from build123d import *

# Parameters (mm, degrees)
F0_W            = 304.8
F0_H            = 106.68
F1_DEPTH        = 3.81
F2_W            = 294.132
F2_H            = 96.012
F3_DEPTH        = 2.54
F4_W            = 5.334
F4_H            = 5.334
F4_W_2          = 5.08
F4_H_2          = 5.08
F5_DEPTH        = 25.4
F6_R            = 5.08
F7_DEPTH        = 27.94
F9_DEPTH        = 27.94
F10_D           = 2.032
F10_DEPTH       = 12.7
F10_CSINK_D     = 3.81
F10_CSINK_ANGLE = 90
F10_TIP         = 0.6104743889


with BuildPart() as f1:
    # F0 (on Top) → F1 (new body)
    with BuildSketch(Plane.XY):
        with Locations((152.4, -53.34)):
            Rectangle(F0_W, F0_H)
    extrude(amount=F1_DEPTH)

    # F2 (on face) → F3 (join)
    with BuildSketch(Plane.XY.offset(3.81)):
        with Locations((152.4, -53.34)):
            Rectangle(F2_W, F2_H)
    extrude(amount=F3_DEPTH)

    # F4 (on face) → F5 (join)
    with BuildSketch(Plane.XY.offset(6.35)):
        with Locations((8.001, -8.001)):
            Rectangle(F4_W, F4_H)
        with Locations((8.001, -98.679)):
            Rectangle(F4_W, F4_H)
        with Locations((296.799, -8.001)):
            Rectangle(F4_W, F4_H)
        with Locations((296.799, -98.679)):
            Rectangle(F4_W, F4_H)
        with Locations((152.4, -7.874)):
            Rectangle(F4_W_2, F4_H_2)
        with Locations((152.4, -98.806)):
            Rectangle(F4_W_2, F4_H_2)
    extrude(amount=F5_DEPTH)

    # F6
    f6_edges = [f1.edges().sort_by_distance(p)[0] for p in [
        (294.132, -96.012, 19.05),
        (294.132, -10.668, 19.05),
        (10.668, -10.668, 19.05),
        (10.668, -96.012, 19.05),
    ]]
    fillet(f6_edges, radius=F6_R)

    # F7 (cut): faces of the model
    f7_faces = [f1.faces().sort_by_distance(p)[0] for p in [
        (7.6306507319, -7.6306507319, 31.75),
        (7.6306507319, -99.0493492681, 31.75),
        (297.1693492681, -7.6306507319, 31.75),
        (297.1693492681, -99.0493492681, 31.75),
    ]]
    extrude(f7_faces, amount=-F7_DEPTH, mode=Mode.SUBTRACT)

    # F9 (cut): faces of the model
    f9_faces = [f1.faces().sort_by_distance(p)[0] for p in [
        (152.4, -7.874, 31.75),
        (152.4, -98.806, 31.75),
    ]]
    extrude(f9_faces, amount=-F9_DEPTH, mode=Mode.SUBTRACT)

    # F10
    with Locations(Plane(origin=(0, 0, 0), x_dir=(1, 0, 0), z_dir=(0, 0, -1))):
        with Locations((3.81, 102.87), (3.81, 3.81), (300.99, 102.87), (300.99, 3.81), (152.4, 3.81), (152.4, 102.87)):
            CounterSinkHole(F10_D / 2, F10_CSINK_D / 2, depth=F10_DEPTH, counter_sink_angle=F10_CSINK_ANGLE)
            with Locations((0, 0, -(F10_DEPTH + F10_TIP / 2))):  # 118° drill point
                Cone(0, F10_D / 2, F10_TIP, mode=Mode.SUBTRACT)


solid = f1.part
Input: part model. Units: mm. Frame: model coordinates. A direction names the side the tool comes from. Give positions to 0.01 mm unless a question says otherwise; leave off trailing zeros. Loops run counter-clockwise (first coordinate to the right, second up) from the corner with the lowest first, then second, coordinate; pieces in that order, holes last. Notation, with made-up numbers: M 51,45.5 L 82,45.5 A26 cw 82,81.5 Z; hole C -36.75,-36.5 d4. An arc over 180 degrees is marked long. Use CSV: the item, a comma, the result in double quotes.
(1) Section B-B, the plane x = 255.5. Return loops of the section in (y, z), plus the area to 3 significant figures.
Outcome:
outline,"M -106.68,0 L 0,0 L 0,3.81 L -5.33,3.81 L -5.33,6.35 L -101.35,6.35 L -101.35,3.81 L -106.68,3.81 Z"
area,"650 mm²"
(2) Pin query (flat end, axial travel): P1, Ø1.3, axis at y = -99, z = 5, coming from the +X side; P2, Ø2, axis at y = -98, z = 5.5, coming from the -X side; P3, Ø1.6, axis at x = 3.81, y = -102.87, coming from the +Z side; P4, Ø3, axis at x = 153.5, z = 5.5, coming from the -Y side. Return the tip coordinate at first contact, or that it passes through.
Outcome:
P1,"stops at x = 294.94"
P2,"stops at x = 8.6"
P3,"passes through"
P4,"stops at y = -101.35"
(3) Section A-A, the plane z = 5. Return loops of the section in (x, y).
Outcome:
outline,"M 5.33,-96.01 L 5.59,-96.01 A5.08 cw 10.67,-101.09 L 10.67,-101.35 L 149.86,-101.35 L 149.86,-96.27 L 154.94,-96.27 L 154.94,-101.35 L 294.13,-101.35 L 294.13,-101.09 A5.08 cw 299.21,-96.01 L 299.47,-96.01 L 299.47,-10.67 L 299.21,-10.67 A5.08 cw 294.13,-5.59 L 294.13,-5.33 L 154.94,-5.33 L 154.94,-10.41 L 149.86,-10.41 L 149.86,-5.33 L 10.67,-5.33 L 10.67,-5.59 A5.08 cw 5.59,-10.67 L 5.33,-10.67 Z"
(4) Material intervals for L1, parallel to X at y = -102.87, z = 2.2; L2, parallel to Y at x = 3.81, z = 1.55; L3, parallel to Y at x = 50, z = 4.75, sorted ascending. Write a range as [from, to].
Outcome:
L1,"x = [0, 2.79], [4.83, 151.38], [153.42, 299.97], [302.01, 304.8]"
L2,"y = [-106.68, -103.89], [-101.85, -4.83], [-2.79, 0]"
L3,"y = [-101.35, -5.33]"
(5) Set-up query: faces 1 (the face through (295.66, -9.22, 5.1)), 2 (the face through (295.58, -97.54, 5.1)), 3 (the face through (9.22, -97.54, 5.1)), 4 (the face through (9.22, -9.14, 5.1)). Return all of +Z, -Z, +X, -X, +Y, -Y with unobstructed straight access to the full face (end or side cutting, diameter ignored); none if empty.
Outcome:
face 1,"+Z, +X, +Y"
face 2,"+Z, +X, -Y"
face 3,"+Z, -X, -Y"
face 4,"+Z, -X, +Y"
